Build history of the part. All positions in model axes, mm. Face numbers are marked on the shaded views. Coordinates: 2 decimals unless noted, no trailing zeros. Loops run counter-clockwise (first coordinate to the right, second up) from the corner with the lowest first, then second, coordinate; pieces in that order, holes last.
(1) Flat gauge pins, fed straight in: P1, Ø3, axis at y = -1, z = -2.5, coming from the +X side; P2, Ø2, axis at y = -1, z = -14.5, coming from the -X side; P3, Ø1, axis at x = 7, z = -11, coming from the -Y side. Where does each tip first touch, or does it go through?
(2) Slice it at A-A (z = 0). Give the cut face in (x, y).
(3) Wall check: L1, parallel to X at y = -4, z = 0; L2, parallel to Y at x = -2.5, z = 9.5; L3, parallel to X at y = -2.45, z = 0.5. Give the ranges that are in metal, low to high.
(4) Two-plate mould, pull along X, no slides. Class the marked faces 1, 2 and 3: pulls with the +X half, pulls with the -X half, needs draft (parallel to the pull), parting line crosses it, or undercut.
(5) Slice it at B-B (x = 0). Give the cut face in (y, z), and give its area (3 significant figures).
(6) Slice it at C-C (y = -3.3). Give the cut face in (x, z), and give its area (3 significant figures).
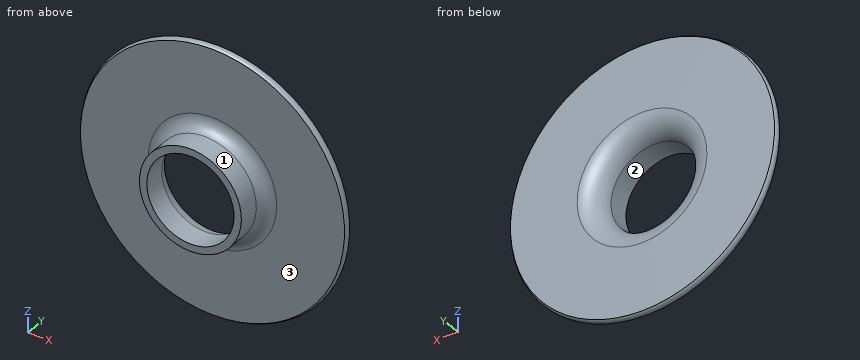
from build123d import *


with BuildPart() as part:
    # Sketch1 → Revolve1 (revolve)
    with BuildSketch(Plane(origin=(0, 0, 0), x_dir=(0, 0, -1), z_dir=(1, 0, 0)), mode=Mode.PRIVATE) as revolve1_sk:
        with BuildLine():
            Line((-18, -1.25), (-8.75, -1.25))
            ThreePointArc((-8.75, -1.25), (-7.600097578, -1.650784896), (-6.94842599, -2.679487115))
            Line((-6.94842599, -2.679487115), (-6.94842599, -5.679487115))
            Line((-6.94842599, -5.679487115), (-5.949317187, -5.679487115))
            Line((-5.949317187, -5.679487115), (-5.949317187, -2.679487115))
            ThreePointArc((-5.949317187, -2.679487115), (-6.941628239, -0.893587174), (-8.847382379, -0.157230615))
            Line((-8.847382379, -0.157230615), (-18, -0.25))
            ThreePointArc((-18, -0.25), (-18.207106781, -0.75), (-18, -1.25))
        make_face()
    revolve(revolve1_sk.sketch.rotate(Axis((0, -237.677688504, 0), (0, 1, 0)), 180), axis=Axis((0, -237.677688504, 0), (0, 1, 0)))


solid = part.part
Response values:
1. P1: stops at x = 18.18
1. P2: stops at x = -12.19
1. P3: stops at y = -1.25
2. outline: (-18, -1.25) - (-8.75, -1.25) arc R1.85 cw to (-6.95, -2.68) - (-6.95, -5.68) - (-5.95, -5.68) - (-5.95, -2.68) arc R3 ccw to (-8.85, -0.16) - (-18, -0.25) arc R0.71 ccw to start; (5.95, -5.68) - (6.95, -5.68) - (6.95, -2.68) arc R1.85 cw to (8.75, -1.25) - (18, -1.25) arc R0.71 ccw to (18, -0.25) - (8.85, -0.16) arc R3 ccw to (5.95, -2.68) - close
3. L1: x = -6.95 to -5.95, 5.95 to 6.95
3. L2: y = -1.25 to -0.17
3. L3: x = -7 to -5.97, 5.97 to 7
4. face 1: parting line crosses it
4. face 2: undercut
4. face 3: needs draft
5. outline: (-5.68, -6.95) - (-2.68, -6.95) arc R1.85 cw to (-1.25, -8.75) - (-1.25, -18) arc R0.71 ccw to (-0.25, -18) - (-0.16, -8.85) arc R3 ccw to (-2.68, -5.95) - (-5.68, -5.95) - close; (-5.68, 5.95) - (-2.68, 5.95) arc R3 ccw to (-0.16, 8.85) - (-0.25, 18) arc R0.71 ccw to (-1.25, 18) - (-1.25, 8.75) arc R1.85 cw to (-2.68, 6.95) - (-5.68, 6.95) - close
5. area: 32.3 mm2
6. outline: circle Ø13.9 at (0, 0); hole circle Ø11.9 at (0, 0)
6. area: 40.5 mm2
